from build123d import *

# Parameters (mm, degrees)
SKETCH_1_W                     = 25
SKETCH_1_H                     = 25
SKETCH_1_W_2                   = 19
SKETCH_1_H_2                   = 19
EXTRUDE_1_DEPTH                = 1207.3
HOLE_WIZARD_7_0_7_1_AT_2_COUNT = 2
HOLE_WIZARD_7_0_7_1_AT_2_PITCH = 70
PATTERN_LINEAR_1_COUNT         = 2
PATTERN_LINEAR_1_PITCH         = 1113.64


with BuildPart() as part:
    # 草图1 → 拉伸1 (new body)
    with BuildSketch(Plane.XY):
        with Locations((12.5, -12.5)):
            Rectangle(SKETCH_1_W, SKETCH_1_H)
        with Locations((12.5, -12.5)):
            Rectangle(SKETCH_1_W_2, SKETCH_1_H_2, mode=Mode.SUBTRACT)
    extrude(amount=EXTRUDE_1_DEPTH)

    # 草图4 → Ø7.0 (7) 直径孔1 (revolve, cut)
    with BuildSketch(Plane(origin=(0, -12.5, 11.8), x_dir=(0, 0, 1), z_dir=(0, 1, 0))):
        Polygon((0, 0), (0, 32.103012167), (3.5, 30), (3.5, 0), align=None)
    hole_wizard_7_0_7_1 = revolve(axis=Axis((-6.35, -12.5, 11.8), (1, 0, 0)), mode=Mode.SUBTRACT)

    # Ø7.0 (7) 直径孔1 at 2: Ø7.0 (7) 直径孔1 ×2
    with Locations(*[(0, 0, i * HOLE_WIZARD_7_0_7_1_AT_2_PITCH) for i in range(1, HOLE_WIZARD_7_0_7_1_AT_2_COUNT)]):
        add(hole_wizard_7_0_7_1, mode=Mode.SUBTRACT)

    # 阵列(线性)1: Ø7.0 (7) 直径孔1 ×2
    with Locations(*[(0, 0, i * PATTERN_LINEAR_1_PITCH) for i in range(1, PATTERN_LINEAR_1_COUNT)]):
        add(hole_wizard_7_0_7_1, mode=Mode.SUBTRACT)

    # 阵列(线性)1 copy 1 sketch → 阵列(线性)1 copy 1 (revolve, cut)
    with BuildSketch(Plane(origin=(0, -12.5, 1195.44), x_dir=(0, 0, 1), z_dir=(0, 1, 0))):
        Polygon((0, 0), (0, 32.103012167), (3.5, 30), (3.5, 0), align=None)
    revolve(axis=Axis((-6.35, -12.5, 1195.44), (1, 0, 0)), mode=Mode.SUBTRACT)


solid = part.part
CAD build for the part. Positions are in the model's coordinates, mm. A direction names the side the tool comes from. Round coordinates to 2 decimals unless told otherwise and drop trailing zeros. Loops run counter-clockwise (first coordinate to the right, second up) from the corner with the lowest first, then second, coordinate; pieces in that order, holes last.
(1) Two-plate mould, pull along Y, no slides. Class faces 1 (the flat face through (3, -13, 595)), 2 (the flat face through (22, -13, 595)), 3 (the flat face through (12, -25, 595)), 4 (the flat face through (23, -12, 0)): +Y half, -Y half, draft (parallel to the pull), parting line (faces both ways), or undercut.
(2) Which spindle directions (+Z, -Z, +X, -X, +Y, -Y) get a long thin tool onto all of the face, cutting with end or side? Do faces 5 (the flat face through (12, -3, 595)), 6 (the flat face through (25, -13, 595)). Say none if no direction does.
(3) Cut at A-A (x = 10.25). Give the cut face in (y, z), plus the area to 3 significant figures.
(4) Wall check: line 1 along Z through (x, y) = (1.05, -12.5); line 2 along X through (y, z) = (-8.75, 439); line 3 along Y through (x, z) = (20.25, 629). Give the ranges that are in metal, low to high.
(5) Drop a flat-ended pin along its axis: pin 1 (3 mm diameter, centred on x = 13.5, y = -6, fed in from -Z). Give the stop position or say it passes through.
(6) Cut at B-B (z = 260). Give the cut face in (x, y).
Findings below:
1. face 1: undercut
1. face 2: undercut
1. face 3: -Y half
1. face 4: draft
2. face 5: +Z, -Z
2. face 6: +Z, -Z, +X, +Y, -Y
3. outline: (-25, 0) - (-22, 0) - (-22, 1207.3) - (-25, 1207.3) - close; (-3, 0) - (0, 0) - (0, 1207.3) - (-3, 1207.3) - close
3. area: 7,240 mm2
4. line 1: z = 0 to 8.3, 15.3 to 78.3, 85.3 to 1121.94, 1128.94 to 1191.94, 1198.94 to 1207.3
4. line 2: x = 0 to 3, 22 to 25
4. line 3: y = -25 to -22, -3 to 0
5. pin 1: passes through
6. outline: (0, -25) - (25, -25) - (25, 0) - (0, 0) - close; hole (3, -22) - (22, -22) - (22, -3) - (3, -3) - close
